Drawing for the job (mm, zero at the part's lowest x, y, z). A direction names the side the tool comes from. Coordinates: 2 decimals unless noted, no trailing zeros. Order: outer loops, then holes, each group sorted by start corner. A loop starts at its lowest first (then second) coordinate and runs counter-clockwise, first axis right, second up. Notation, with made-up numbers: (12, 66.25) -> (71, 66.25) arc R32 cw to (71, 98.25) -> close; hole circle Ø1 at (29, -25.5). An arc over 180 degrees is marked (long way). Write each question's results on one line, items separated by ' | '.
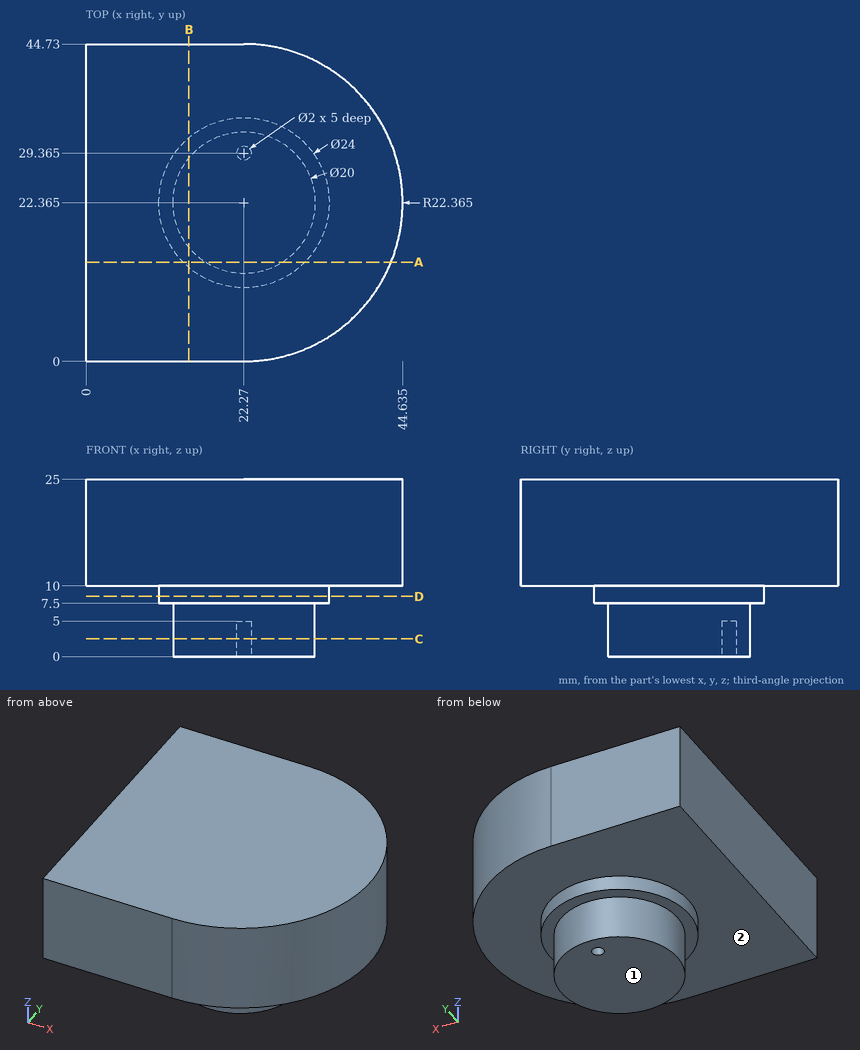
Item 1: Drill centre lines: line 1 (Z direction, x = 3, y = 7.5); line 2 (Y direction, x = 22.27, z = 2.4) (3 decimals); line 3 (X direction, y = 3.5, z = 11). Where is each one in solid material? Low to high. Write a range as from..to.
Answer:
line 1: z = 10..25 | line 2: y = 12.365..28.365, 30.365..32.365 | line 3: x = 0..34.28
Item 2: Slice it at D-D, the plane z = 8.5. List the corners of the cut face in (x, y) (3 decimals).
Answer:
outline: circle Ø24 at (22.27, 22.365)
Item 3: Pin check, flat tips, straight feed: pin 1 (1 mm diameter, centred on x = 24.5, z = 9, fed in from +Y); pin 2 (1 mm diameter, centred on x = 5, y = 36.5, fed in from -Z); pin 3 (2 mm diameter, centred on y = 27.5, z = 5, fed in from -X). Stop position of each tip, or through.
Answer:
pin 1: stops at y = 34.24 | pin 2: stops at z = 10 | pin 3: stops at x = 13.16
Item 4: Slice it at C-C, the plane z = 2.5. List the corners of the cut face in (x, y) (3 decimals), and give its area (3 significant figures).
Answer:
outline: circle Ø20 at (22.27, 22.365); hole circle Ø2 at (22.27, 29.365) | area: 311 mm^2
Item 5: Tool access for the marked faces 1 and 2: list every direction of +Z, -Z, +X, -X, +Y, -Y with a clear straight run to the whole face (end or side of a thin tool).
Answer:
face 1: -Z, +X, -X, +Y, -Y | face 2: -Z
Item 6: Slice it at A-A, the plane y = 14. List the corners of the cut face in (x, z).
Answer:
outline: (0, 10) -> (13.67, 10) -> (13.67, 7.5) -> (16.79, 7.5) -> (16.79, 0) -> (27.75, 0) -> (27.75, 7.5) -> (30.87, 7.5) -> (30.87, 10) -> (43.01, 10) -> (43.01, 25) -> (0, 25) -> close
Item 7: Slice it at B-B, the plane x = 14.5. List the corners of the cut face in (y, z), and give its area (3 significant figures).
Answer:
outline: (0, 10) -> (13.22, 10) -> (13.22, 7.5) -> (16.07, 7.5) -> (16.07, 0) -> (28.66, 0) -> (28.66, 7.5) -> (31.51, 7.5) -> (31.51, 10) -> (44.73, 10) -> (44.73, 25) -> (0, 25) -> close | area: 811 mm^2
